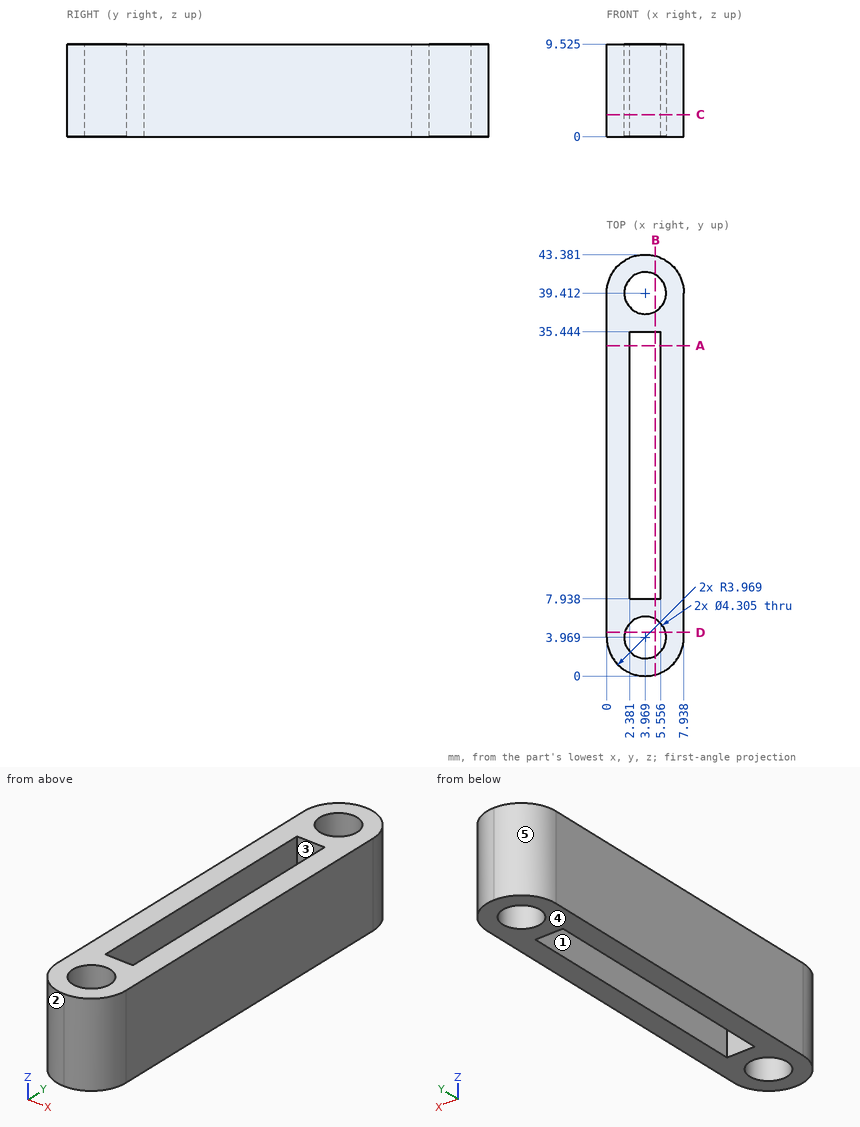
For this review, use the dimensioned drawing (mm, ordinates from the lowest corner) and the shaded views. A direction names the side the tool comes from. Round coordinates to 2 decimals unless told otherwise and drop trailing zeros. Write each loop counter-clockwise with the first axis right and the second up, starting at its lowest first coordinate (ties: lowest second). Pieces come first, ordered by that corner, then holes. Notation, with made-up numbers: M 39,63 L 49,63 A10 ccw 49,81 Z; hole C 17.25,69 d4. An arc over 180 degrees is marked long. Answer as CSV lines item,"result". Start each with the question number.
Q1. Wall thickness on line 1 along X through (y, z) = (16.5, 8); line 2 along Y through (x, z) = (3.75, 7.75) (1 decimal); line 3 along Y through (x, z) = (4.25, 5) (1 decimal): over which ranges is each line inside the solid? List them lowest first.
Q2. Consider section C-C, the plane z = 2.25. State how many separate pieces and enclosed holes the cut face has.
Q3. Consider section D-D, the plane y = 4.5. Give the boundary of the cut face in (x, z) (1 decimal).
Q4. Tool access review of the marked faces 1 and 2: name each direction out of +Z, -Z, +X, -X, +Y, -Y from which nothing blocks a thin tool from reaching the whole face with its end or side.
Q5. Consider section B-B, the plane x = 5. Give the boundary of the cut face in (y, z) (1 decimal).
Q6. Consider section A-A, the plane y = 34. Give the boundary of the cut face in (x, z) (1 decimal).
Q7. The part is to be moulded in two halves that separate along Y. For the marked faces 3, 4 and 5, say which applies: +Y half, -Y half, draft (parallel to the pull), parting line (faces both ways), or undercut.
Q8. Clearance check with flat-ended pins moving along their axes: P1, Ø2, axis at x = 7, z = 7, coming from the -Y side; P2, Ø1.5, axis at x = 5, z = 6.5, coming from the -Y side. State where each tip first meets the part, or that it passes through.
Result set:
1,line 1,"x = 0 to 2.38, 5.56 to 7.94"
1,line 2,"y = 0 to 1.8, 6.1 to 7.9, 35.4 to 37.3, 41.6 to 43.4"
1,line 3,"y = 0 to 1.8, 6.1 to 7.9, 35.4 to 37.3, 41.5 to 43.4"
2,separate pieces,"1"
2,enclosed holes,"3"
3,outline,"M 0,0 L 1.9,0 L 1.9,9.5 L 0,9.5 Z; M 6.1,0 L 7.9,0 L 7.9,9.5 L 6.1,9.5 Z"
4,face 1,"+Z, -Z"
4,face 2,"+Z, -Z, -X, -Y"
5,outline,"M 0.1,0 L 2.1,0 L 2.1,9.5 L 0.1,9.5 Z; M 5.9,0 L 7.9,0 L 7.9,9.5 L 5.9,9.5 Z; M 35.4,0 L 37.5,0 L 37.5,9.5 L 35.4,9.5 Z; M 41.3,0 L 43.2,0 L 43.2,9.5 L 41.3,9.5 Z"
6,outline,"M 0,0 L 2.4,0 L 2.4,9.5 L 0,9.5 Z; M 5.6,0 L 7.9,0 L 7.9,9.5 L 5.6,9.5 Z"
7,face 3,"undercut"
7,face 4,"draft"
7,face 5,"+Y half"
8,P1,"stops at y = 0.56"
8,P2,"stops at y = 0.01"
